For this review, use the dimensioned drawing (mm, ordinates from the lowest corner) and the shaded views. Coordinates: 2 decimals unless noted, no trailing zeros. Loops run counter-clockwise (first coordinate to the right, second up) from the corner with the lowest first, then second, coordinate; pieces in that order, holes last.
1. Mouldability with a two-part tool opening along Y and no side actions: class the marked faces 1, 2 and 3 as pulls with the +Y half, pulls with the -Y half, needs draft (parallel to the pull), parting line crosses it, or undercut.
2. To check wall thickness, follow probe 1 along Y at (x, z) = (12.5, 34); probe 2 along Y at (x, z) = (3, 28.5); probe 3 along Z at (x, y) = (4.25, 41.5). State the ranges of each line that lie inside material, in increasing order.
3. Clearance check with flat-ended pins moving along their axes: P1, Ø4, axis at x = 15.5, y = 15, coming from the +Z side; P2, Ø1, axis at x = 8.5, y = 25.5, coming from the +Z side; P3, Ø2, axis at x = 6, z = 43.5, coming from the +Y side. State where each tip first meets the part, or that it passes through.
4. Take a section at C-C, the plane x = 12.5. State the section outline as (y, z) points.
5. Take a section at A-A, the plane z = 34. State the section outline as (x, y) points.
6. Take a section at D-D, the plane x = 19. State the section outline as (y, z) points.
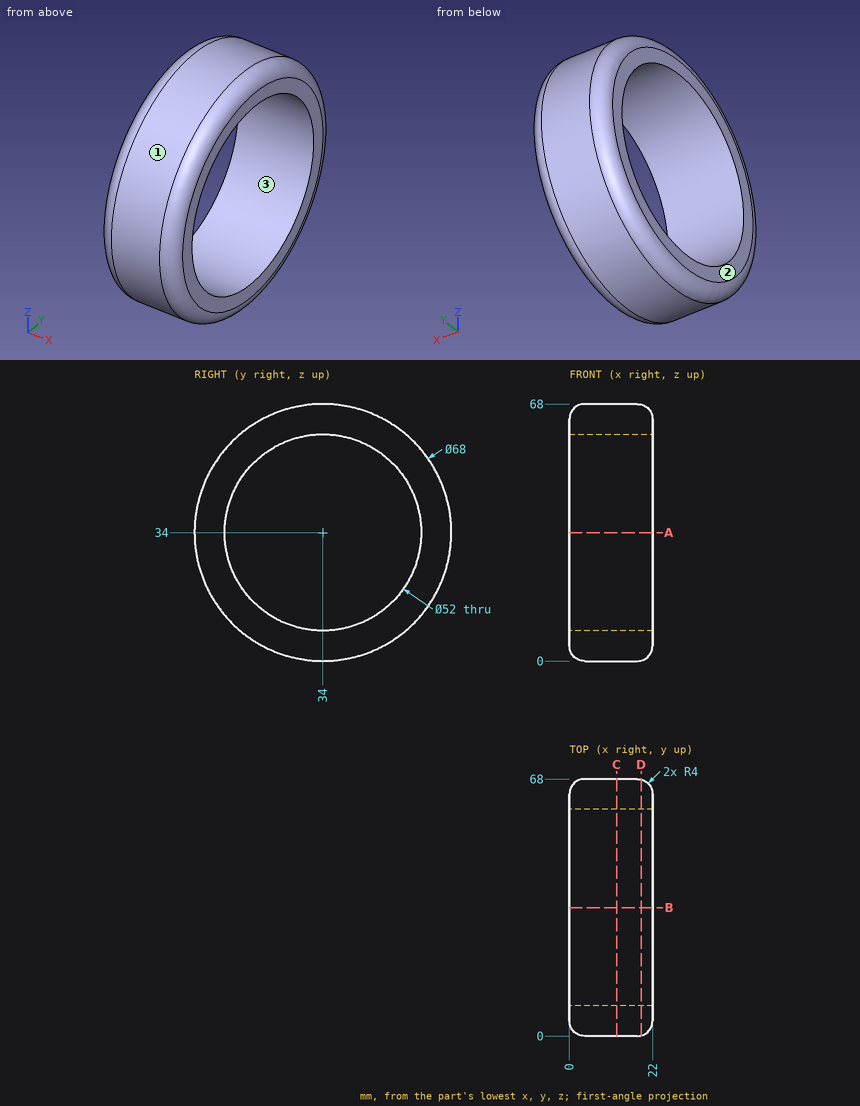
Results list:
1. face 1: parting line crosses it
1. face 2: needs draft
1. face 3: undercut
2. probe 1: y = 0 to 8, 60 to 68
2. probe 2: y = 0.58 to 8.59, 59.41 to 67.42
2. probe 3: z = 0.84 to 9.11, 58.89 to 67.16
3. P1: stops at z = 63.44
3. P2: stops at z = 67.05
3. P3: stops at y = 66.92
4. outline: circle Ø68 at (34, 34); hole circle Ø52 at (34, 34)
5. outline: (0, 4) arc R4 ccw to (4, 0) - (18, 0) arc R4 ccw to (22, 4) - (22, 8) - (0, 8) - close; (0, 60) - (22, 60) - (22, 64) arc R4 ccw to (18, 68) - (4, 68) arc R4 ccw to (0, 64) - close
6. outline: circle Ø67.75 at (34, 34); hole circle Ø52 at (34, 34)
